from build123d import *

# Parameters (mm, degrees)
ESBO_O1_W                = 35
ESBO_O1_H                = 28
RESSALTO_EXTRUS_O1_DEPTH = 30
ESBO_O2_R                = 5.15
CORTE_EXTRUS_O1_DEPTH    = 31
ESBO_O3_R                = 11
CORTE_EXTRUS_O2_DEPTH    = 4
ESBO_O4_R                = 1.5
CORTE_EXTRUS_O3_DEPTH    = 10
ESBO_O6_R                = 2
CORTE_EXTRUS_O4_DEPTH    = 7


with BuildPart() as part:
    # Esboço1 → Ressalto-extrusão1 (new body)
    with BuildSketch(Plane.XY):
        Rectangle(ESBO_O1_W, ESBO_O1_H)
    extrude(amount=RESSALTO_EXTRUS_O1_DEPTH)

    # Esboço2 → Corte-extrusão1 (cut, through all)
    with BuildSketch(Plane.XY.offset(30)):
        Circle(ESBO_O2_R)
    extrude(amount=-CORTE_EXTRUS_O1_DEPTH, mode=Mode.SUBTRACT)

    # Esboço3 → Corte-extrusão2 (cut)
    with BuildSketch(Plane.XY.offset(30)):
        Circle(ESBO_O3_R)
    extrude(amount=-CORTE_EXTRUS_O2_DEPTH, mode=Mode.SUBTRACT)

    # Esboço4 → Corte-extrusão3 (cut)
    with BuildSketch(Plane.XY.offset(26)):
        with Locations((-8, 0)):
            Circle(ESBO_O4_R)
        with Locations((8, 0)):
            Circle(ESBO_O4_R)
    extrude(amount=-CORTE_EXTRUS_O3_DEPTH, mode=Mode.SUBTRACT)

    # Esboço6 → Corte-extrusão4 (cut)
    with BuildSketch(Plane(origin=(0, 14, 0), x_dir=(1, 0, 0), z_dir=(0, 1, 0))):
        with Locations((-12, -24)):
            Circle(ESBO_O6_R)
        with Locations((12, -24)):
            Circle(ESBO_O6_R)
        with Locations((12, -6)):
            Circle(ESBO_O6_R)
        with Locations((-12, -6)):
            Circle(ESBO_O6_R)
    extrude(amount=-CORTE_EXTRUS_O4_DEPTH, mode=Mode.SUBTRACT)


solid = part.part
Read the model definition and answer for the solid it produces. Units are mm, in the model's axes. A direction names the side the tool comes from. Give positions to 0.01 mm unless a question says otherwise; leave off trailing zeros. Write each loop counter-clockwise with the first axis right and the second up, starting at its lowest first coordinate (ties: lowest second). Pieces come first, ordered by that corner, then holes. Notation, with made-up numbers: M 10,51.25 L 44,51.25 A7 cw 44,64.25 Z; hole C -39,-37.5 d4. An arc over 180 degrees is marked long. One line per item, written item: value. Start each with the question number.
(1) Find section B-B (x = -12). Determine the outline of the cut face in (y, z).
(2) Determine the mould class of faces 1 (the cylindrical face through (10, 11, 24)), 2 (the flat face through (0, -14, 15)), 3 (the flat face through (-8, 0, 16)) for opening direction Z: pulls with the +Z half, pulls with the -Z half, needs draft (parallel to the pull), parting line crosses it, or undercut.
(3) Find the intervals of material crossed by line 1 (X direction, y = 12.25, z = 6); line 2 (Z direction, x = -12, y = 10); line 3 (Y direction, x = 8, z = 17.25), in increasing order.
(4) Find section A-A (z = 24). Determine the outline of the cut face in (x, y).
(5) Find section D-D (x = 3). Determine the outline of the cut face in (y, z), plus the area to 3 significant figures.
(6) Flat-ended cylindrical pins translate along their axes: pin 1 Ø3 at (x, z) = (-12, 6) entering from +Y; pin 2 Ø5 at (x, y) = (8, 0) entering from +Z. Find the tip coordinate at first contact, or state that the pin passes through.
(7) A tool of negligible diameter and unlimited length cuts with its end or side. For faces 4 (the flat face through (8, 0, 16)), 5 (the flat face through (-12, 7, 6)), 6 (the cylindrical face through (4.91, 1.55, 13.18)), from which of +Z, -Z, +X, -X, +Y, -Y can it reach the whole face along a straight path? Write none if from no direction.
(8) Find section C-C (y = 0). Determine the outline of the cut face in (x, z).
Results below:
1. outline: M -14,0 L 14,0 L 14,4 L 7,4 L 7,8 L 14,8 L 14,22 L 7,22 L 7,26 L 14,26 L 14,30 L -14,30 Z
2. face 1: undercut
2. face 2: needs draft
2. face 3: pulls with the +Z half
3. line 1: x = -17.5 to -14, -10 to 10, 14 to 17.5
3. line 2: z = 0 to 4, 8 to 22, 26 to 30
3. line 3: y = -14 to -1.5, 1.5 to 14
4. outline: M -17.5,-14 L 17.5,-14 L 17.5,14 L 14,14 L 14,7 L 10,7 L 10,14 L -10,14 L -10,7 L -14,7 L -14,14 L -17.5,14 Z; hole C -8,0 d3; hole C 0,0 d10.3; hole C 8,0 d3
5. outline: M -14,0 L -4.19,0 L -4.19,26 L -10.58,26 L -10.58,30 L -14,30 Z; M 4.19,0 L 14,0 L 14,30 L 10.58,30 L 10.58,26 L 4.19,26 Z
5. area: 538 mm^2
6. pin 1: stops at y = 7
6. pin 2: stops at z = 26
7. face 4: +Z
7. face 5: +Y
7. face 6: +Z, -Z
8. outline: M -17.5,0 L -5.15,0 L -5.15,26 L -6.5,26 L -6.5,16 L -9.5,16 L -9.5,26 L -11,26 L -11,30 L -17.5,30 Z; M 5.15,0 L 17.5,0 L 17.5,30 L 11,30 L 11,26 L 9.5,26 L 9.5,16 L 6.5,16 L 6.5,26 L 5.15,26 Z
